from build123d import *

# Parameters (mm, degrees)
SKETCH1_R           = 4
SKETCH1_R_2         = 1.5
SKETCH1_R_3         = 2
BOSS_EXTRUDE1_DEPTH = 2
SKETCH2_W           = 42
SKETCH2_H           = 2
SKETCH2_W_2         = 8.75
BOSS_EXTRUDE2_DEPTH = 23.4
FILLET1_R           = 2
FILLET2_R           = 2
CUT_EXTRUDE1_REACH  = 73.172
SKETCH3_R           = 2
CUT_EXTRUDE2_REACH  = 75.085
SKETCH4_R           = 1.5


with BuildPart() as part:
    # Sketch1 → Boss-Extrude1 (new body)
    with BuildSketch(Plane(origin=(0, 0, 0), x_dir=(1, 0, 0), z_dir=(0, 1, 0))):
        with BuildLine():
            Line((0, 4), (0, 25.5))
            ThreePointArc((0, 25.5), (0.878679656, 27.621320344), (3, 28.5))
            Line((3, 28.5), (8, 28.5))
            Line((8, 28.5), (8, 36.5))
            Line((8, 36.5), (50, 36.5))
            Line((50, 36.5), (50, 28.5))
            Line((50, 28.5), (55, 28.5))
            ThreePointArc((55, 28.5), (57.121320344, 27.621320344), (58, 25.5))
            Line((58, 25.5), (58, 4))
            Line((58, 4), (49.25, 4))
            Line((49.25, 4), (49.25, 9.5))
            Line((49.25, 9.5), (47.1, 9.5))
            Line((47.1, 9.5), (47.1, 3))
            ThreePointArc((47.1, 3), (46.221320344, 0.878679656), (44.1, 0))
            Line((44.1, 0), (13.9, 0))
            ThreePointArc((13.9, 0), (11.778679656, 0.878679656), (10.9, 3))
            Line((10.9, 3), (10.9, 9.5))
            Line((10.9, 9.5), (8.75, 9.5))
            Line((8.75, 9.5), (8.75, 4))
            Line((8.75, 4), (0, 4))
        make_face()
        with Locations(Location((39.5, 12.3, 0), (0, 0, 270))):
            Circle(SKETCH1_R, mode=Mode.SUBTRACT)
        with Locations(Location((18.5, 12.3, 0), (0, 0, 90))):
            Circle(SKETCH1_R, mode=Mode.SUBTRACT)
        with Locations(Location((18.5, 19.4, 0), (0, 0, 270))):
            Circle(SKETCH1_R_2, mode=Mode.SUBTRACT)
        with Locations(Location((39.5, 19.4, 0), (0, 0, 270))):
            Circle(SKETCH1_R_2, mode=Mode.SUBTRACT)
        with Locations(Location((46.6, 12.3, 0), (0, 0, 270))):
            Circle(SKETCH1_R_2, mode=Mode.SUBTRACT)
        with Locations(Location((39.5, 5.2, 0), (0, 0, 270))):
            Circle(SKETCH1_R_2, mode=Mode.SUBTRACT)
        with Locations(Location((32.4, 12.3, 0), (0, 0, 270))):
            Circle(SKETCH1_R_2, mode=Mode.SUBTRACT)
        with Locations(Location((25.6, 12.3, 0), (0, 0, 270))):
            Circle(SKETCH1_R_2, mode=Mode.SUBTRACT)
        with Locations(Location((18.5, 5.2, 0), (0, 0, 270))):
            Circle(SKETCH1_R_2, mode=Mode.SUBTRACT)
        with Locations(Location((11.4, 12.3, 0), (0, 0, 270))):
            Circle(SKETCH1_R_2, mode=Mode.SUBTRACT)
        with Locations(Location((29, 23, 0), (0, 0, 270))):
            Circle(SKETCH1_R, mode=Mode.SUBTRACT)
        with Locations(Location((29, 30.1, 0), (0, 0, 270))):
            Circle(SKETCH1_R_2, mode=Mode.SUBTRACT)
        with Locations(Location((36.1, 23, 0), (0, 0, 270))):
            Circle(SKETCH1_R_2, mode=Mode.SUBTRACT)
        with Locations(Location((29, 15.9, 0), (0, 0, 270))):
            Circle(SKETCH1_R_2, mode=Mode.SUBTRACT)
        with Locations(Location((21.9, 23, 0), (0, 0, 270))):
            Circle(SKETCH1_R_2, mode=Mode.SUBTRACT)
        with Locations(Location((53, 22.5, 0), (0, 0, 270))):
            Circle(SKETCH1_R_3, mode=Mode.SUBTRACT)
        with Locations(Location((5, 22.5, 0), (0, 0, 90))):
            Circle(SKETCH1_R_3, mode=Mode.SUBTRACT)
        with Locations(Location((53, 12.5, 0), (0, 0, 270))):
            Circle(SKETCH1_R_3, mode=Mode.SUBTRACT)
        with Locations(Location((5, 12.5, 0), (0, 0, 90))):
            Circle(SKETCH1_R_3, mode=Mode.SUBTRACT)
    extrude(amount=BOSS_EXTRUDE1_DEPTH)

    # Sketch2 → Boss-Extrude2 (add)
    with BuildSketch(Plane(origin=(0, 2, 0), x_dir=(1, 0, 0), z_dir=(0, 1, 0))):
        with Locations((29, 35.5)):
            Rectangle(SKETCH2_W, SKETCH2_H)
        with Locations((4.375, 5)):
            Rectangle(SKETCH2_W_2, SKETCH2_H)
        with Locations((53.625, 5)):
            Rectangle(SKETCH2_W_2, SKETCH2_H)
    extrude(amount=BOSS_EXTRUDE2_DEPTH)

    # Fillet1
    fillet1_edges = [part.edges().sort_by_distance(p)[0] for p in [
        (8, 25.4, -35.5),
        (50, 25.4, -35.5),
        (0, 25.4, -5),
        (8.75, 25.4, -5),
        (49.25, 25.4, -5),
        (58, 25.4, -5),
    ]]
    fillet(fillet1_edges, radius=FILLET1_R)

    # Fillet2
    fillet2_edges = [part.edges().sort_by_distance(p)[0] for p in [
        (53.625, 0, -4),
        (4.375, 0, -4),
        (29, 0, -36.5),
    ]]
    fillet(fillet2_edges, radius=FILLET2_R)

    # Sketch3 → Cut-Extrude1 (cut, up to next)
    with BuildSketch(Plane.XY.offset(-4), mode=Mode.PRIVATE) as cut_extrude1_sk1:
        with Locations((5, 19.05)):
            Circle(SKETCH3_R)
    cut_extrude1_tool1 = extrude(cut_extrude1_sk1.sketch, amount=-CUT_EXTRUDE1_REACH, mode=Mode.PRIVATE) & part.part
    # Sketch3 → Cut-Extrude1 (cut, up to next)
    with BuildSketch(Plane.XY.offset(-4), mode=Mode.PRIVATE) as cut_extrude1_sk2:
        with Locations((5, 9.05)):
            Circle(SKETCH3_R)
    cut_extrude1_tool2 = extrude(cut_extrude1_sk2.sketch, amount=-CUT_EXTRUDE1_REACH, mode=Mode.PRIVATE) & part.part
    # Sketch3 → Cut-Extrude1 (cut, up to next)
    with BuildSketch(Plane.XY.offset(-4), mode=Mode.PRIVATE) as cut_extrude1_sk3:
        with Locations((53, 9.05)):
            Circle(SKETCH3_R)
    cut_extrude1_tool3 = extrude(cut_extrude1_sk3.sketch, amount=-CUT_EXTRUDE1_REACH, mode=Mode.PRIVATE) & part.part
    # Sketch3 → Cut-Extrude1 (cut, up to next)
    with BuildSketch(Plane.XY.offset(-4), mode=Mode.PRIVATE) as cut_extrude1_sk4:
        with Locations((53, 19.05)):
            Circle(SKETCH3_R)
    cut_extrude1_tool4 = extrude(cut_extrude1_sk4.sketch, amount=-CUT_EXTRUDE1_REACH, mode=Mode.PRIVATE) & part.part
    add(cut_extrude1_tool1.solids().sort_by_distance((5, 19.05, -4))[0], mode=Mode.SUBTRACT)
    add(cut_extrude1_tool2.solids().sort_by_distance((5, 9.05, -4))[0], mode=Mode.SUBTRACT)
    add(cut_extrude1_tool3.solids().sort_by_distance((53, 9.05, -4))[0], mode=Mode.SUBTRACT)
    add(cut_extrude1_tool4.solids().sort_by_distance((53, 19.05, -4))[0], mode=Mode.SUBTRACT)

    # Sketch4 → Cut-Extrude2 (cut, up to next)
    with BuildSketch(Plane(origin=(0, 0, -36.5), x_dir=(-1, 0, 0), z_dir=(0, 0, -1)), mode=Mode.PRIVATE) as cut_extrude2_sk1:
        with Locations((-18.65, 13.4)):
            Circle(SKETCH4_R)
    cut_extrude2_tool1 = extrude(cut_extrude2_sk1.sketch, amount=-CUT_EXTRUDE2_REACH, mode=Mode.PRIVATE) & part.part
    # Sketch4 → Cut-Extrude2 (cut, up to next)
    with BuildSketch(Plane(origin=(0, 0, -36.5), x_dir=(-1, 0, 0), z_dir=(0, 0, -1)), mode=Mode.PRIVATE) as cut_extrude2_sk2:
        with Locations((-18.65, 20.4)):
            Circle(SKETCH4_R)
    cut_extrude2_tool2 = extrude(cut_extrude2_sk2.sketch, amount=-CUT_EXTRUDE2_REACH, mode=Mode.PRIVATE) & part.part
    # Sketch4 → Cut-Extrude2 (cut, up to next)
    with BuildSketch(Plane(origin=(0, 0, -36.5), x_dir=(-1, 0, 0), z_dir=(0, 0, -1)), mode=Mode.PRIVATE) as cut_extrude2_sk3:
        with Locations((-11.65, 13.4)):
            Circle(SKETCH4_R)
    cut_extrude2_tool3 = extrude(cut_extrude2_sk3.sketch, amount=-CUT_EXTRUDE2_REACH, mode=Mode.PRIVATE) & part.part
    # Sketch4 → Cut-Extrude2 (cut, up to next)
    with BuildSketch(Plane(origin=(0, 0, -36.5), x_dir=(-1, 0, 0), z_dir=(0, 0, -1)), mode=Mode.PRIVATE) as cut_extrude2_sk4:
        with Locations((-18.65, 6.4)):
            Circle(SKETCH4_R)
    cut_extrude2_tool4 = extrude(cut_extrude2_sk4.sketch, amount=-CUT_EXTRUDE2_REACH, mode=Mode.PRIVATE) & part.part
    # Sketch4 → Cut-Extrude2 (cut, up to next)
    with BuildSketch(Plane(origin=(0, 0, -36.5), x_dir=(-1, 0, 0), z_dir=(0, 0, -1)), mode=Mode.PRIVATE) as cut_extrude2_sk5:
        with Locations((-25.65, 13.4)):
            Circle(SKETCH4_R)
    cut_extrude2_tool5 = extrude(cut_extrude2_sk5.sketch, amount=-CUT_EXTRUDE2_REACH, mode=Mode.PRIVATE) & part.part
    # Sketch4 → Cut-Extrude2 (cut, up to next)
    with BuildSketch(Plane(origin=(0, 0, -36.5), x_dir=(-1, 0, 0), z_dir=(0, 0, -1)), mode=Mode.PRIVATE) as cut_extrude2_sk6:
        with Locations((-39.35, 6.4)):
            Circle(SKETCH4_R)
    cut_extrude2_tool6 = extrude(cut_extrude2_sk6.sketch, amount=-CUT_EXTRUDE2_REACH, mode=Mode.PRIVATE) & part.part
    # Sketch4 → Cut-Extrude2 (cut, up to next)
    with BuildSketch(Plane(origin=(0, 0, -36.5), x_dir=(-1, 0, 0), z_dir=(0, 0, -1)), mode=Mode.PRIVATE) as cut_extrude2_sk7:
        with Locations((-46.35, 13.4)):
            Circle(SKETCH4_R)
    cut_extrude2_tool7 = extrude(cut_extrude2_sk7.sketch, amount=-CUT_EXTRUDE2_REACH, mode=Mode.PRIVATE) & part.part
    # Sketch4 → Cut-Extrude2 (cut, up to next)
    with BuildSketch(Plane(origin=(0, 0, -36.5), x_dir=(-1, 0, 0), z_dir=(0, 0, -1)), mode=Mode.PRIVATE) as cut_extrude2_sk8:
        with Locations((-39.35, 13.4)):
            Circle(SKETCH4_R)
    cut_extrude2_tool8 = extrude(cut_extrude2_sk8.sketch, amount=-CUT_EXTRUDE2_REACH, mode=Mode.PRIVATE) & part.part
    # Sketch4 → Cut-Extrude2 (cut, up to next)
    with BuildSketch(Plane(origin=(0, 0, -36.5), x_dir=(-1, 0, 0), z_dir=(0, 0, -1)), mode=Mode.PRIVATE) as cut_extrude2_sk9:
        with Locations((-39.35, 20.4)):
            Circle(SKETCH4_R)
    cut_extrude2_tool9 = extrude(cut_extrude2_sk9.sketch, amount=-CUT_EXTRUDE2_REACH, mode=Mode.PRIVATE) & part.part
    # Sketch4 → Cut-Extrude2 (cut, up to next)
    with BuildSketch(Plane(origin=(0, 0, -36.5), x_dir=(-1, 0, 0), z_dir=(0, 0, -1)), mode=Mode.PRIVATE) as cut_extrude2_sk10:
        with Locations((-32.35, 13.4)):
            Circle(SKETCH4_R)
    cut_extrude2_tool10 = extrude(cut_extrude2_sk10.sketch, amount=-CUT_EXTRUDE2_REACH, mode=Mode.PRIVATE) & part.part
    add(cut_extrude2_tool1.solids().sort_by_distance((18.65, 13.4, -36.5))[0], mode=Mode.SUBTRACT)
    add(cut_extrude2_tool2.solids().sort_by_distance((18.65, 20.4, -36.5))[0], mode=Mode.SUBTRACT)
    add(cut_extrude2_tool3.solids().sort_by_distance((11.65, 13.4, -36.5))[0], mode=Mode.SUBTRACT)
    add(cut_extrude2_tool4.solids().sort_by_distance((18.65, 6.4, -36.5))[0], mode=Mode.SUBTRACT)
    add(cut_extrude2_tool5.solids().sort_by_distance((25.65, 13.4, -36.5))[0], mode=Mode.SUBTRACT)
    add(cut_extrude2_tool6.solids().sort_by_distance((39.35, 6.4, -36.5))[0], mode=Mode.SUBTRACT)
    add(cut_extrude2_tool7.solids().sort_by_distance((46.35, 13.4, -36.5))[0], mode=Mode.SUBTRACT)
    add(cut_extrude2_tool8.solids().sort_by_distance((39.35, 13.4, -36.5))[0], mode=Mode.SUBTRACT)
    add(cut_extrude2_tool9.solids().sort_by_distance((39.35, 20.4, -36.5))[0], mode=Mode.SUBTRACT)
    add(cut_extrude2_tool10.solids().sort_by_distance((32.35, 13.4, -36.5))[0], mode=Mode.SUBTRACT)


solid = part.part
Work out the finished part from the listing and answer in its coordinate system (mm). A direction names the side the tool comes from. Round coordinates to 2 decimals unless told otherwise and drop trailing zeros. Order: outer loops, then holes, each group sorted by start corner. A loop starts at its lowest first (then second) coordinate and runs counter-clockwise, first axis right, second up. Notation, with made-up numbers: M 24,21 L 75,21 A17 cw 75,40 Z; hole C -30,36 d7. An arc over 180 degrees is marked long. Put each result on its own line as item: value. Start each with the question number.
Q1. Flat-ended cylindrical pins translate along their axes: pin 1 (0.6 mm diameter, centred on x = 52.5, y = 1, fed in from -Z); pin 2 (1.6 mm diameter, centred on x = 48, y = 1, fed in from +Z); pin 3 (7 mm diameter, centred on x = 53.5, y = 19.5, fed in from +Z). Find the tip coordinate at first contact, or state that the pin passes through.
Q2. Straight lines are drawn through the part: L1, parallel to X at y = 1.55, z = -5.2; L2, parallel to Y at x = 39.35, z = -36; L3, parallel to Z at x = 12.5, y = 8.75. For each, find the intervals that lie inside material, in ascending order. Write a range as [from, to].
Q3. For a pull along X with two mould halves and no side action, classify faces 4 (the cylindrical face through (3, 19, -5)), 5 (the cylindrical face through (29.29, 0.6, -35.93)), 6 (the flat face through (58, 6, -5)) as pulls with the +X half, pulls with the -X half, needs draft (parallel to the pull), parting line crosses it, or undercut.
Q4. Section D-D, the plane y = 3.25 is taken. Write down the section's boundary in (x, z).
Q5. Section C-C, the plane z = -5.2 is taken. Give the number of separate pieces and of enclosed holes in the cut face, and give its area (3 significant figures).
Q6. A tool of negligible diameter and unlimited length cuts with its end or side. For faces 1 (the flat face through (10.9, 1, -6)), 2 (the cylindrical face through (8.57, 24.8, -35.51)), 3 (the flat face through (5, 1, -28.5)), from which of +Z, -Z, +X, -X, +Y, -Y can it reach the whole face along a straight path? Write none if from no direction.
Q7. Section A-A, the plane y = 9.05 is taken. Write down the section's boundary in (x, z).
Q8. Section B-B, the plane z = -30.1 is taken. Write down the section's boundary in (x, y), and give its area (3 significant figures).
Findings below:
1. pin 1: stops at z = -28.5
1. pin 2: stops at z = -9.5
1. pin 3: stops at z = -4
2. L1: x = [0, 8.75], [10.9, 17], [20, 38], [41, 47.1], [49.25, 58]
2. L2: y = [0.68, 4.9], [7.9, 11.9], [14.9, 18.9], [21.9, 25.4]
2. L3: z = [-36.5, -34.5]
3. face 4: undercut
3. face 5: needs draft
3. face 6: pulls with the +X half
4. outline: M 0,-6 L 8.75,-6 L 8.75,-4 L 0,-4 Z; M 8,-36.5 L 50,-36.5 L 50,-34.5 L 8,-34.5 Z; M 49.25,-6 L 58,-6 L 58,-4 L 49.25,-4 Z
5. separate pieces: 5
5. enclosed holes: 4
5. area: 448 mm^2
6. face 1: +Z, +Y, -Y
6. face 2: -Z, -X, +Y
6. face 3: -Z, -X, +Y, -Y
7. outline: M 0,-6 L 3,-6 L 3,-4 L 0,-4 Z; M 7,-6 L 8.75,-6 L 8.75,-4 L 7,-4 Z; M 8,-36.5 L 50,-36.5 L 50,-34.5 L 8,-34.5 Z; M 49.25,-6 L 51,-6 L 51,-4 L 49.25,-4 Z; M 55,-6 L 58,-6 L 58,-4 L 55,-4 Z
8. outline: M 8,0 L 27.5,0 L 27.5,2 L 8,2 Z; M 30.5,0 L 50,0 L 50,2 L 30.5,2 Z
8. area: 78.0 mm^2
